```python
from build123d import *

# Parameters (mm, degrees)
SKETCH_1_R          = 20
EXTRUDE_1_DEPTH     = 4
SKETCH_2_R          = 1
CUT_EXTRUDE_1_DEPTH = 4


with BuildPart() as part:
    # Эскиз1 → Бобышка-Вытянуть1 (new body)
    with BuildSketch(Plane.XY):
        Circle(SKETCH_1_R)
    extrude(amount=EXTRUDE_1_DEPTH)

    # Эскиз2 → Вырез-Вытянуть1 (cut)
    with BuildSketch(Plane.XY.offset(4)):
        with Locations((0, 5)):
            Circle(SKETCH_2_R)
        with Locations((0, -5)):
            Circle(SKETCH_2_R)
        with BuildLine():
            Line((-1.58113883, 2.25), (1.58113883, 2.25))
            ThreePointArc((1.58113883, 2.25), (2.75, 0), (1.58113883, -2.25))
            Line((1.58113883, -2.25), (-1.58113883, -2.25))
            ThreePointArc((-1.58113883, -2.25), (-2.75, 0), (-1.58113883, 2.25))
        make_face()
    extrude(amount=-CUT_EXTRUDE_1_DEPTH, mode=Mode.SUBTRACT)


solid = part.part
```
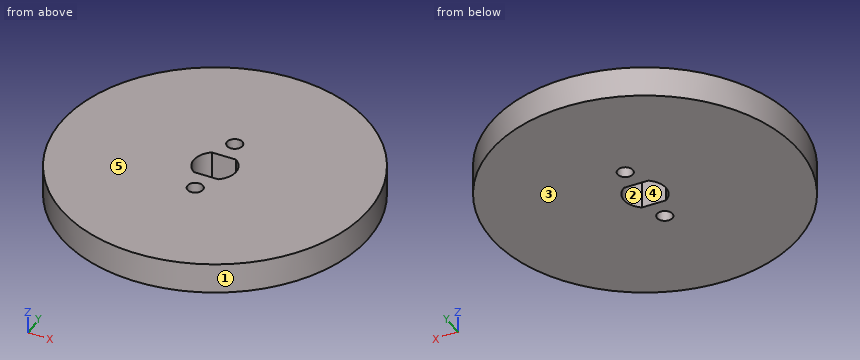
Work out the finished part from the listing and answer in its coordinate system (mm). Face numbers are marked on the shaded views. A direction names the side the tool comes from. Coordinates: 2 decimals unless noted, no trailing zeros. Order: outer loops, then holes, each group sorted by start corner. A loop starts at its lowest first (then second) coordinate and runs counter-clockwise, first axis right, second up. Notation, with made-up numbers: (-16.75, 58.5) - (12.25, 58.5) arc R20 ccw to (12.25, 90.5) - close; hole circle Ø4 at (0.25, 11). An arc over 180 degrees is marked (long way). Answer as a JSON object with one key per item and string values.
1. Find section C-C on z = 3.25. Determine the outline of the cut face in (x, y).
Output values:
{"outline": "circle Ø40 at (0, 0); hole (-1.58, -2.25) - (1.58, -2.25) arc R2.75 ccw to (1.58, 2.25) - (-1.58, 2.25) arc R2.75 ccw to start; hole circle Ø2 at (0, -5); hole circle Ø2 at (0, 5)"}
2. A tool of negligible diameter and unlimited length cuts with its end or side. For the marked faces 4 and 5, from which of +Z, -Z, +X, -X, +Y, -Y can it reach the whole face along a straight path? Write none if from no direction.
Output values:
{"face 4": "+Z, -Z", "face 5": "+Z, +X, -X, +Y, -Y"}
3. Find section A-A on x = 0. Determine the outline of the cut face in (y, z).
Output values:
{"outline": "(-20, 0) - (-6, 0) - (-6, 4) - (-20, 4) - close; (-4, 0) - (-2.25, 0) - (-2.25, 4) - (-4, 4) - close; (2.25, 0) - (4, 0) - (4, 4) - (2.25, 4) - close; (6, 0) - (20, 0) - (20, 4) - (6, 4) - close"}
4. Consider line 1 (Y direction, x = 0, z = 2.55); line 2 (X direction, y = 2, z = 0.2); line 3 (X direction, y = 14, z = 0.3). Determine where each line is inside the solid, lowest interval first.
Output values:
{"line 1": "y = -20 to -6, -4 to -2.25, 2.25 to 4, 6 to 20", "line 2": "x = -19.9 to -1.89, 1.89 to 19.9", "line 3": "x = -14.28 to 14.28"}
5. Find section D-D on y = 5. Determine the outline of the cut face in (x, z).
Output values:
{"outline": "(-19.36, 0) - (-1, 0) - (-1, 4) - (-19.36, 4) - close; (1, 0) - (19.36, 0) - (19.36, 4) - (1, 4) - close"}
6. Find section B-B on y = 0. Determine the outline of the cut face in (x, z), plus the area to 3 significant figures.
Output values:
{"outline": "(-20, 0) - (-2.75, 0) - (-2.75, 4) - (-20, 4) - close; (2.75, 0) - (20, 0) - (20, 4) - (2.75, 4) - close", "area": "138 mm²"}
7. Each of these flat-tipped pins is pushed along its axis until it touches: P1, Ø2, axis at x = -7, z = 3, coming from the +Y side; P2, Ø0.9, axis at x = -0.5, z = 2, coming from the -Y side; P3, Ø1.5, axis at x = -4.5, y = -4.5, coming from the -Z side; P4, Ø2, axis at x = -12.5, z = 2.5, coming from the +Y side. Where does it stop, or does it pass through?
Output values:
{"P1": "stops at y = 19.08", "P2": "stops at y = -20", "P3": "stops at z = 0", "P4": "stops at y = 16.36"}
8. The mould has two halves that part along X. Classify the marked faces 1, 2 and 3: +X half, -X half, draft (parallel to the pull), parting line (faces both ways), or undercut.
Output values:
{"face 1": "parting line", "face 2": "undercut", "face 3": "draft"}
